Geometry check sheet. Reference: the model listing, model coordinates, mm. A direction names the side the tool comes from. Coordinates: 2 decimals unless noted, no trailing zeros. Loops run counter-clockwise (first coordinate to the right, second up) from the corner with the lowest first, then second, coordinate; pieces in that order, holes last. Notation, with made-up numbers: M -15,36.5 L -1,36.5 A7 cw -1,43.5 Z; hole C 50,33.5 d7. An arc over 180 degrees is marked long. Use CSV: the item, a comma, the result in double quotes.
```python
from build123d import *

# Parameters (mm, degrees)
SKETCH1_R           = 3
BOSS_EXTRUDE1_DEPTH = 20
SKETCH8_W           = 105
SKETCH8_H           = 12.5
CUT_EXTRUDE7_DEPTH  = 8
SKETCH9_W           = 105
SKETCH9_H           = 12.5
CUT_EXTRUDE8_DEPTH  = 8


with BuildPart() as part:
    # Sketch1 → Boss-Extrude1 (new body)
    with BuildSketch(Plane(origin=(0, 0, 0), x_dir=(1, 0, 0), z_dir=(0, 1, 0))):
        with BuildLine():
            Line((-20, 30), (97.83, 30))
            Line((97.83, 30), (97.83, 10))
            Line((97.83, 10), (21.160500507, 10))
            Line((21.160500507, 10), (15, 0))
            ThreePointArc((15, 0), (-1.903014387, -14.878794852), (-14.517138166, 3.775274755))
            ThreePointArc((-14.517138166, 3.775274755), (-15.852441132, 8.126182851), (-20, 10))
            ThreePointArc((-20, 10), (-30, 20), (-20, 30))
        make_face()
        Circle(SKETCH1_R, mode=Mode.SUBTRACT)
    extrude(amount=BOSS_EXTRUDE1_DEPTH)

    # Sketch8 → Cut-Extrude7 (cut)
    with BuildSketch(Plane.XZ):
        with Locations((33.915, -20.25)):
            Rectangle(SKETCH8_W, SKETCH8_H)
    extrude(amount=-CUT_EXTRUDE7_DEPTH, mode=Mode.SUBTRACT)

    # Sketch9 → Cut-Extrude8 (cut)
    with BuildSketch(Plane(origin=(0, 20, 0), x_dir=(1, 0, 0), z_dir=(0, 1, 0))):
        with Locations((33.915, 20)):
            Rectangle(SKETCH9_W, SKETCH9_H)
    extrude(amount=-CUT_EXTRUDE8_DEPTH, mode=Mode.SUBTRACT)


solid = part.part
```
1. Release check for a two-part mould opening along X. For faces 1 (the flat face through (18.123, 9.86, -5.07)), 2 (the flat face through (38, 10, -30)), 3 (the flat face through (33, 8, -20)) record: +X half, -X half, draft (parallel to the pull), parting line (faces both ways), or undercut.
The answers:
face 1,"+X half"
face 2,"draft"
face 3,"undercut"
2. Section check A-A, the plane x = 0. Record the cut outline in (y, z), plus the area to 3 significant figures.
The answers:
outline,"M 0,-30 L 20,-30 L 20,-26.25 L 12,-26.25 L 12,-13.75 L 20,-13.75 L 20,-3 L 0,-3 L 0,-14 L 8,-14 L 8,-26.5 L 0,-26.5 Z; M 0,3 L 20,3 L 20,15 L 0,15 Z"
area,"580 mm^2"
3. Section check D-D, the plane y = 4.5. Record the cut outline in (x, z) (1 decimal).
The answers:
outline,"M -20,-30 L 97.8,-30 L 97.8,-10 L 21.2,-10 L 15,0 A15 ccw long -14.5,-3.8 A5.5 cw -20,-10 A10 ccw Z; hole M -18.6,-26.5 L 86.4,-26.5 L 86.4,-14 L -18.6,-14 Z; hole C 0,0 d6"
4. Gauge pin test, flat ends, axial feed: P1, Ø1, axis at x = 67, y = 8.5, coming from the +Z side; P2, Ø5, axis at x = 5, z = -17, coming from the +Y side; P3, Ø10, axis at y = 11, z = 0, coming from the +X side. Record the tip position at first contact, or that the pin passes through.
The answers:
P1,"z = -10"
P2,"y = 12"
P3,"x = 18.08"
5. Section check B-B, the plane z = -20. Record the cut outline in (x, y) (3 decimals).
The answers:
outline,"M -30,0 L -18.585,0 L -18.585,8 L 86.415,8 L 86.415,0 L 97.83,0 L 97.83,20 L 86.415,20 L 86.415,12 L -18.585,12 L -18.585,20 L -30,20 Z"
6. Set-up check for faces 4 (the flat face through (33, 12, -20)), 5 (the flat face through (-18.585, 4, -20)), 6 (the cylindrical face through (-3, 10, 0)), 7 (the flat face through (21, 0, -13)), 8 (the cylindrical face through (-15.81, 9.86, -8.08)): record each of +Z, -Z, +X, -X, +Y, -Y from which the full face is reachable in a straight line by a thin tool's end or side.
The answers:
face 4,"+Y"
face 5,"-Y"
face 6,"+Y, -Y"
face 7,"+Z, -Z, +X, -X, -Y"
face 8,"-X, +Y, -Y"
7. Thickness scan on line 1 (Z direction, x = 0, y = 12.75); line 2 (Z direction, x = 0, y = 4.5); line 3 (Z direction, x = 41, y = 7.5). Record the ranges inside material, lowest first. Write a range as [from, to].
The answers:
line 1,"[-30, -26.25], [-13.75, -3], [3, 15]"
line 2,"[-30, -26.5], [-14, -3], [3, 15]"
line 3,"[-30, -26.5], [-14, -10]"
8. Section check C-C, the plane x = 69.5. Record the cut outline in (y, z).
The answers:
outline,"M 0,-30 L 20,-30 L 20,-26.25 L 12,-26.25 L 12,-13.75 L 20,-13.75 L 20,-10 L 0,-10 L 0,-14 L 8,-14 L 8,-26.5 L 0,-26.5 Z"
